from build123d import *
from build123d.topology import SkipClean

# Parameters (mm, degrees)
BOSS_EXTRUDE2_DEPTH = 76.2
SCALE2_SCALE        = 0.039370079
BOSS_EXTRUDE3_DEPTH = 3
SKETCH4_R           = 5
SKETCH4_R_2         = 1.5
BOSS_EXTRUDE5_DEPTH = 2
CUT_EXTRUDE1_START  = -29
CUT_EXTRUDE1_DEPTH  = 29


with BuildPart() as part:
    # Sketch1 → Boss-Extrude2 (new body)
    with BuildSketch(Plane(origin=(0, 0, 0), x_dir=(1, 0, 0), z_dir=(0, 1, 0))):
        with BuildLine():
            Line((-38.1, 127), (0, 127))
            Line((0, 127), (0, 254))
            Line((0, 254), (406.4, 254))
            Line((406.4, 254), (406.4, 127))
            Line((406.4, 127), (444.5, 127))
            ThreePointArc((444.5, 127), (482.6, 165.1), (520.7, 127))
            Line((520.7, 127), (647.7, 127))
            ThreePointArc((647.7, 127), (685.8, 165.1), (723.9, 127))
            Line((723.9, 127), (762, 127))
            Line((762, 127), (762, 254))
            Line((762, 254), (1168.4, 254))
            Line((1168.4, 254), (1168.4, 127))
            Line((1168.4, 127), (1206.5, 127))
            ThreePointArc((1206.5, 127), (1244.6, 165.1), (1282.7, 127))
            Line((1282.7, 127), (1346.2, 127))
            Line((1346.2, 127), (1346.2, 381))
            Line((1346.2, 381), (-177.8, 381))
            Line((-177.8, 381), (-177.8, 127))
            Line((-177.8, 127), (-114.3, 127))
            ThreePointArc((-114.3, 127), (-76.2, 165.1), (-38.1, 127))
        make_face()
        with BuildLine():
            Line((0, 0), (0, 127))
            Line((0, 127), (-38.1, 127))
            ThreePointArc((-38.1, 127), (-76.2, 88.9), (-114.3, 127))
            Line((-114.3, 127), (-177.8, 127))
            Line((-177.8, 127), (-177.8, -127))
            Line((-177.8, -127), (1346.2, -127))
            Line((1346.2, -127), (1346.2, 127))
            Line((1346.2, 127), (1282.7, 127))
            ThreePointArc((1282.7, 127), (1244.6, 88.9), (1206.5, 127))
            Line((1206.5, 127), (1168.4, 127))
            Line((1168.4, 127), (1168.4, 0))
            Line((1168.4, 0), (762, 0))
            Line((762, 0), (762, 127))
            Line((762, 127), (723.9, 127))
            ThreePointArc((723.9, 127), (685.8, 88.9), (647.7, 127))
            Line((647.7, 127), (520.7, 127))
            ThreePointArc((520.7, 127), (482.6, 88.9), (444.5, 127))
            Line((444.5, 127), (406.4, 127))
            Line((406.4, 127), (406.4, 0))
            Line((406.4, 0), (0, 0))
        make_face()
    extrude(amount=BOSS_EXTRUDE2_DEPTH)


with BuildPart() as part_1:
    # Scale2: scaled about (584.2, 38.1, -127)
    add(part.part.scale(SCALE2_SCALE).moved(Location((561.2, 36.6, -122))))

    # Sketch3 → Boss-Extrude3 (add)
    # profile 1 of 3: a face of its own
    with BuildSketch(Plane.XY.offset(-117)):
        Polygon((564.2, 49.6), (554.2, 49.6), (554.2, 39.6), (584.2, 39.6), (614.2, 39.6), (614.2, 49.6), (604.2, 49.6), align=None)
        with BuildLine():
            ThreePointArc((585.7, 44.6), (585.260660172, 43.539339828), (584.2, 43.1))
            ThreePointArc((584.2, 43.1), (583.139339828, 45.660660172), (585.7, 44.6))
        make_face(mode=Mode.SUBTRACT)
    # profile 2 of 3: a face of its own
    with BuildSketch(Plane.XY.offset(-117)):
        Polygon((554.2, 59.6), (554.2, 49.6), (564.2, 49.6), (564.2, 59.6), (559.2, 59.6), align=None)
        with BuildLine():
            ThreePointArc((560.7, 54.6), (558.139339828, 53.539339828), (559.2, 56.1))
            ThreePointArc((559.2, 56.1), (560.260660172, 55.660660172), (560.7, 54.6))
        make_face(mode=Mode.SUBTRACT)
    # profile 3 of 3: a face of its own
    with BuildSketch(Plane.XY.offset(-117)):
        Polygon((604.2, 59.6), (604.2, 49.6), (614.2, 49.6), (614.2, 59.6), (609.2, 59.6), align=None)
        with BuildLine():
            ThreePointArc((610.7, 54.6), (608.139339828, 53.539339828), (609.2, 56.1))
            ThreePointArc((609.2, 56.1), (610.260660172, 55.660660172), (610.7, 54.6))
        make_face(mode=Mode.SUBTRACT)
    extrude(amount=-BOSS_EXTRUDE3_DEPTH)

    # Sketch4 → Boss-Extrude5 (add)
    # profile 1 of 2: a face of its own
    with BuildSketch(Plane(origin=(0, 0, -120), x_dir=(-1, 0, 0), z_dir=(0, 0, -1))):
        with Locations((-559.2, 54.6)):
            Circle(SKETCH4_R)
        with Locations(Location((-559.2, 54.6, 0), (0, 0, 180))):
            Circle(SKETCH4_R_2, mode=Mode.SUBTRACT)
    # profile 2 of 2: a face of its own
    with BuildSketch(Plane(origin=(0, 0, -120), x_dir=(-1, 0, 0), z_dir=(0, 0, -1))):
        with Locations((-609.2, 54.6)):
            Circle(SKETCH4_R)
        with Locations(Location((-609.2, 54.6, 0), (0, 0, 180))):
            Circle(SKETCH4_R_2, mode=Mode.SUBTRACT)
    extrude(amount=BOSS_EXTRUDE5_DEPTH)

    # Sketch5 → Cut-Extrude1 (cut)
    with SkipClean():  # the faces are left unmerged after this step: merging them gives an invalid solid
        with BuildSketch(Plane(origin=(0, 0, -122), x_dir=(-1, 0, 0), z_dir=(0, 0, -1)).offset(CUT_EXTRUDE1_START)):
            with BuildLine():
                ThreePointArc((-614.2, 54.6), (-612.735533906, 58.135533906), (-609.2, 59.6))
                Line((-609.2, 59.6), (-614.2, 59.6))
                Line((-614.2, 59.6), (-614.2, 54.6))
            make_face()
            with BuildLine():
                Line((-604.2, 59.6), (-609.2, 59.6))
                ThreePointArc((-609.2, 59.6), (-605.664466094, 58.135533906), (-604.2, 54.6))
                Line((-604.2, 54.6), (-604.2, 59.6))
            make_face()
            with BuildLine():
                ThreePointArc((-564.2, 54.6), (-562.735533906, 58.135533906), (-559.2, 59.6))
                Line((-559.2, 59.6), (-564.2, 59.6))
                Line((-564.2, 59.6), (-564.2, 54.6))
            make_face()
            with BuildLine():
                Line((-554.2, 59.6), (-559.2, 59.6))
                ThreePointArc((-559.2, 59.6), (-555.664466094, 58.135533906), (-554.2, 54.6))
                Line((-554.2, 54.6), (-554.2, 59.6))
            make_face()
        extrude(amount=CUT_EXTRUDE1_DEPTH, mode=Mode.SUBTRACT)
    add(part_1.part.scale(1), mode=Mode.REPLACE)  # the faces are merged on a copy


solid = part_1.part
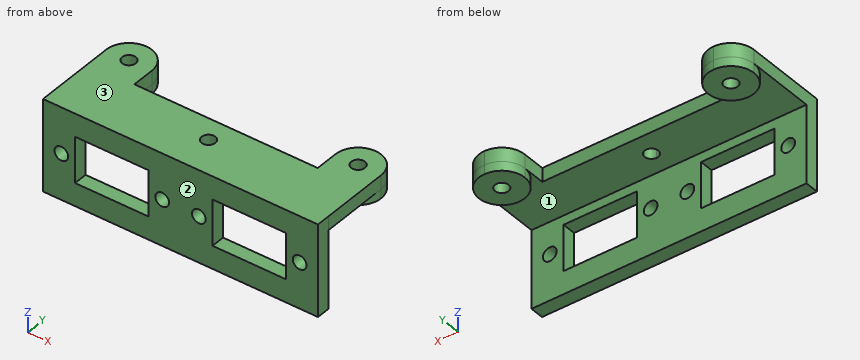
The listing builds one solid part. Answer for the finished solid, in the listing's coordinates (mm). Face numbers are marked on the shaded views. Round coordinates to 2 decimals unless told otherwise and drop trailing zeros. Write each loop counter-clockwise with the first axis right and the second up, starting at its lowest first coordinate (ties: lowest second). Pieces come first, ordered by that corner, then holes. Notation, with made-up numbers: (77.25, 34) - (128.25, 34) arc R11 ccw to (128.25, 51) - close; hole circle Ø6 at (-27.5, 59). An arc over 180 degrees is marked (long way). Use a Markdown table: item, result. Add a question column.
1. For a pull along Y with two mould halves and no side action, classify the marked faces 1, 2 and 3 as +Y half, -Y half, draft (parallel to the pull), parting line (faces both ways), or undercut.
2. The part is cut by section A-A (z = -127). Write down the section's boundary in (x, y).
3. The part is cut by section D-D (x = 589). Write down the section's boundary in (y, z), and give its area (3 significant figures).
4. The part is cut by section B-B (x = 572.5). Write down the section's boundary in (y, z), and give its area (3 significant figures).
5. The part is cut by section C-C (y = 43.75). Write down the section's boundary in (x, z), and give its area (3 significant figures).
6. Consider line 1 (X direction, y = 54.6, z = -120.65); line 2 (Y direction, x = 559.2, z = -119.35); line 3 (X direction, y = 54, z = -118.5). Determine where each line is inside the solid, lowest interval first.
7. Flat-ended cylindrical pins translate along their axes: P1, Ø8, axis at x = 608, y = 53.5, coming from the -Z side; P2, Ø2, axis at x = 607.5, z = -130, coming from the +Y side; P3, Ø0.9, axis at x = 581.5, z = -118.5, coming from the +Y side. Find the tip coordinate at first contact, or state that the pin passes through.
Reported:
| question | item | result |
|---|---|---|
| 1 | face 1 | undercut |
| 1 | face 2 | -Y half |
| 1 | face 3 | draft |
| 2 | outline | (554.2, 36.6) - (556.7, 36.6) - (556.7, 39.6) - (554.2, 39.6) - close; (559.7, 36.6) - (561.2, 36.6) - (561.2, 39.6) - (559.7, 39.6) - close; (577.2, 36.6) - (578.7, 36.6) - (578.7, 39.6) - (577.2, 39.6) - close; (581.7, 36.6) - (586.7, 36.6) - (586.7, 39.6) - (581.7, 39.6) - close; (589.7, 36.6) - (591.2, 36.6) - (591.2, 39.6) - (589.7, 39.6) - close; (607.2, 36.6) - (608.7, 36.6) - (608.7, 39.6) - (607.2, 39.6) - close; (611.7, 36.6) - (614.2, 36.6) - (614.2, 39.6) - (611.7, 39.6) - close |
| 3 | outline | (36.6, -137) - (39.6, -137) - (39.6, -128.27) - (36.6, -128.27) - close; (36.6, -125.73) - (39.6, -125.73) - (39.6, -120) - (49.6, -120) - (49.6, -117) - (36.6, -117) - close |
| 3 | area | 82.4 mm^2 |
| 4 | outline | (36.6, -137) - (39.6, -137) - (39.6, -132) - (36.6, -132) - close; (36.6, -122) - (39.6, -122) - (39.6, -120) - (49.6, -120) - (49.6, -117) - (36.6, -117) - close |
| 4 | area | 60.0 mm^2 |
| 5 | outline | (554.2, -120) - (582.96, -120) - (582.96, -117) - (554.2, -117) - close; (585.44, -120) - (614.2, -120) - (614.2, -117) - (585.44, -117) - close |
| 5 | area | 173 mm^2 |
| 6 | line 1 | 554.2 to 557.7, 560.7 to 564.2, 604.2 to 607.7, 610.7 to 614.2 |
| 6 | line 2 | 36.6 to 53.1, 56.1 to 59.6 |
| 6 | line 3 | 554.2 to 557.83, 560.57 to 564.2, 604.2 to 607.83, 610.57 to 614.2 |
| 7 | P1 | z = -122 |
| 7 | P2 | y = 39.6 |
| 7 | P3 | y = 49.6 |
